Design review of the part shown in the three views and the two pictorial views. Dimensions are in mm from the part's minimum x, y and z. A direction names the side the tool comes from. Round coordinates to 2 decimals unless told otherwise and drop trailing zeros. Order: outer loops, then holes, each group sorted by start corner. A loop starts at its lowest first (then second) coordinate and runs counter-clockwise, first axis right, second up. Notation, with made-up numbers: M 59.5,3 L 95.5,3 A15 ccw 95.5,19 Z; hole C 39,45 d5. An arc over 180 degrees is marked long. Use a Markdown table: item, result. Add a question column.
(1) The part is to be moulded in two halves that separate along Y. For the marked faces 4, 5, 6 and 7, say which applies: released by +Y, released by -Y, zero draft, split by the parting line, or undercut.
(2) Take a section at D-D (x = 44.3). Write out the cut boundary in (y, z), then the cut area to 3 significant figures.
(3) Machinability: for the marked faces 1, 2 and 3, which of the approach directions +Z, -Z, +X, -X, +Y, -Y give a long, thin tool a straight path to every point of the face, cutting with its end or side? Answer none if there is none.
(4) For pin 1 (14 mm diameter, centred on x = 48, z = 14.5, fed in from +Y); pin 2 (1.5 mm diameter, centred on x = 5, z = 5.5, fed in from -Y); pin 3 (6 mm diameter, centred on x = 28.5, z = 40, fed in from -Y); pin 4 (13 mm diameter, centred on x = 37.5, z = 27.5, fed in from -Y), all flat-tipped, find the tip position at first contact; note any pin that passes through.
(5) To check wall thickness, follow probe 1 along Z at (x, y) = (5.9, 7.5); probe 2 along Y at (x, z) = (3, 28.5); probe 3 along Z at (x, y) = (3, 18). State the ranges of each line that lie inside material, in increasing order. Write a range as from..to.
(6) Take a section at B-B (z = 10). Write out the cut boundary in (x, y), then the cut area to 3 significant figures.
(7) Take a section at C-C (y = 15). Write out the cut boundary in (x, z), then the cut area to 3 significant figures.
(8) Take a section at A-A (x = 5.9). Write out the cut boundary in (y, z), then the cut area to 3 significant figures.
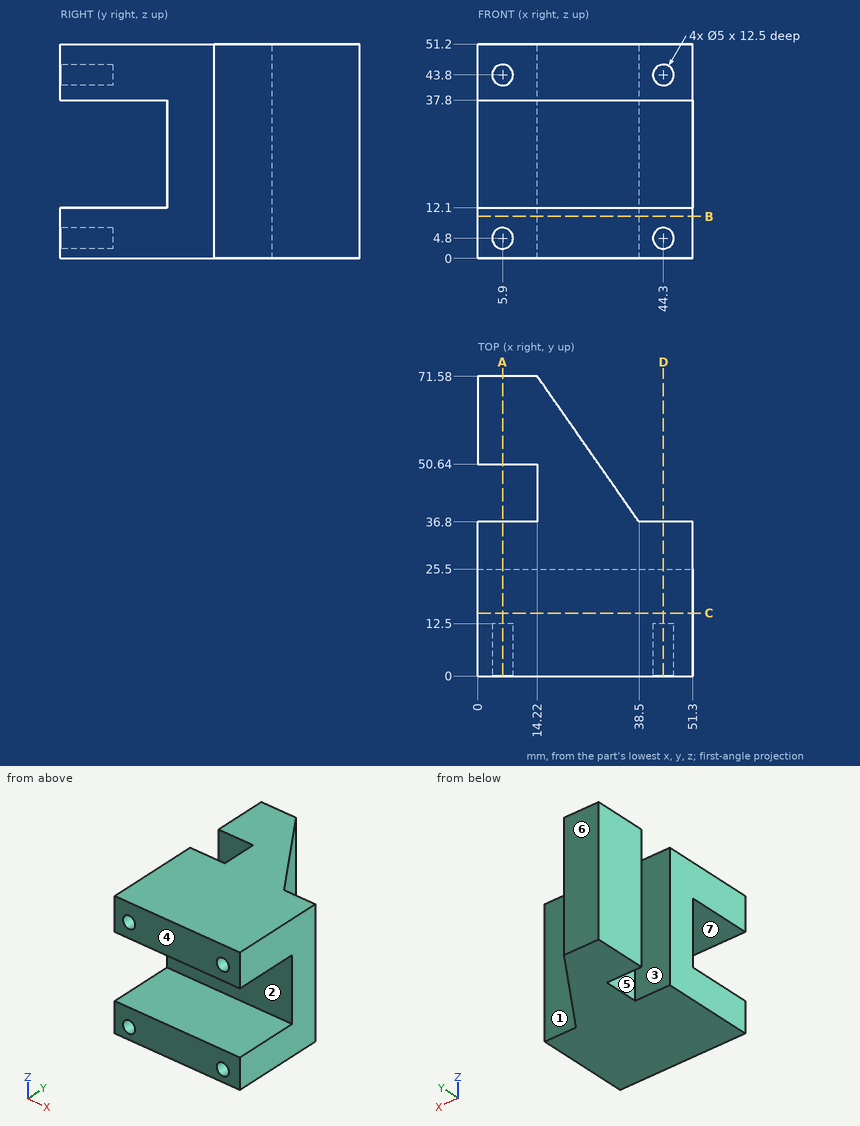
Verdict:
| question | item | result |
|---|---|---|
| 1 | face 4 | released by -Y |
| 1 | face 5 | undercut |
| 1 | face 6 | released by +Y |
| 1 | face 7 | zero draft |
| 2 | outline | M 0,0 L 36.8,0 L 36.8,51.2 L 0,51.2 L 0,46.3 L 12.5,46.3 L 12.5,41.3 L 0,41.3 L 0,37.8 L 25.5,37.8 L 25.5,12.1 L 0,12.1 L 0,7.3 L 12.5,7.3 L 12.5,2.3 L 0,2.3 Z |
| 2 | area | 1,100 mm^2 |
| 3 | face 1 | +Z, -Z, +X, +Y |
| 3 | face 2 | +X, -X, -Y |
| 3 | face 3 | +Z, -Z, -X |
| 4 | pin 1 | stops at y = 36.8 |
| 4 | pin 2 | stops at y = 12.5 |
| 4 | pin 3 | stops at y = 0 |
| 4 | pin 4 | stops at y = 25.5 |
| 5 | probe 1 | z = 0..2.3, 7.3..12.1, 37.8..41.3, 46.3..51.2 |
| 5 | probe 2 | y = 25.5..36.8, 50.64..71.58 |
| 5 | probe 3 | z = 0..12.1, 37.8..51.2 |
| 6 | outline | M 0,0 L 51.3,0 L 51.3,36.8 L 38.5,36.8 L 14.22,71.58 L 0,71.58 L 0,50.64 L 14.22,50.64 L 14.22,36.8 L 0,36.8 Z |
| 6 | area | 2,610 mm^2 |
| 7 | outline | M 0,0 L 51.3,0 L 51.3,12.1 L 0,12.1 Z; M 0,37.8 L 51.3,37.8 L 51.3,51.2 L 0,51.2 Z |
| 7 | area | 1,310 mm^2 |
| 8 | outline | M 0,0 L 36.8,0 L 36.8,51.2 L 0,51.2 L 0,46.3 L 12.5,46.3 L 12.5,41.3 L 0,41.3 L 0,37.8 L 25.5,37.8 L 25.5,12.1 L 0,12.1 L 0,7.3 L 12.5,7.3 L 12.5,2.3 L 0,2.3 Z; M 50.64,0 L 71.58,0 L 71.58,51.2 L 50.64,51.2 Z |
| 8 | area | 2,180 mm^2 |
